Design review of the part shown in the three views and the two pictorial views. Dimensions are in mm from the part's minimum x, y and z. Give positions to 0.01 mm unless a question says otherwise; leave off trailing zeros. Order: outer loops, then holes, each group sorted by start corner. A loop starts at its lowest first (then second) coordinate and runs counter-clockwise, first axis right, second up. Notation, with made-up numbers: (20, 71.5) - (75, 71.5) arc R30 cw to (75, 103.5) - close; hole circle Ø9 at (36.5, 45.25). An arc over 180 degrees is marked (long way). Put each result on its own line as item: value.
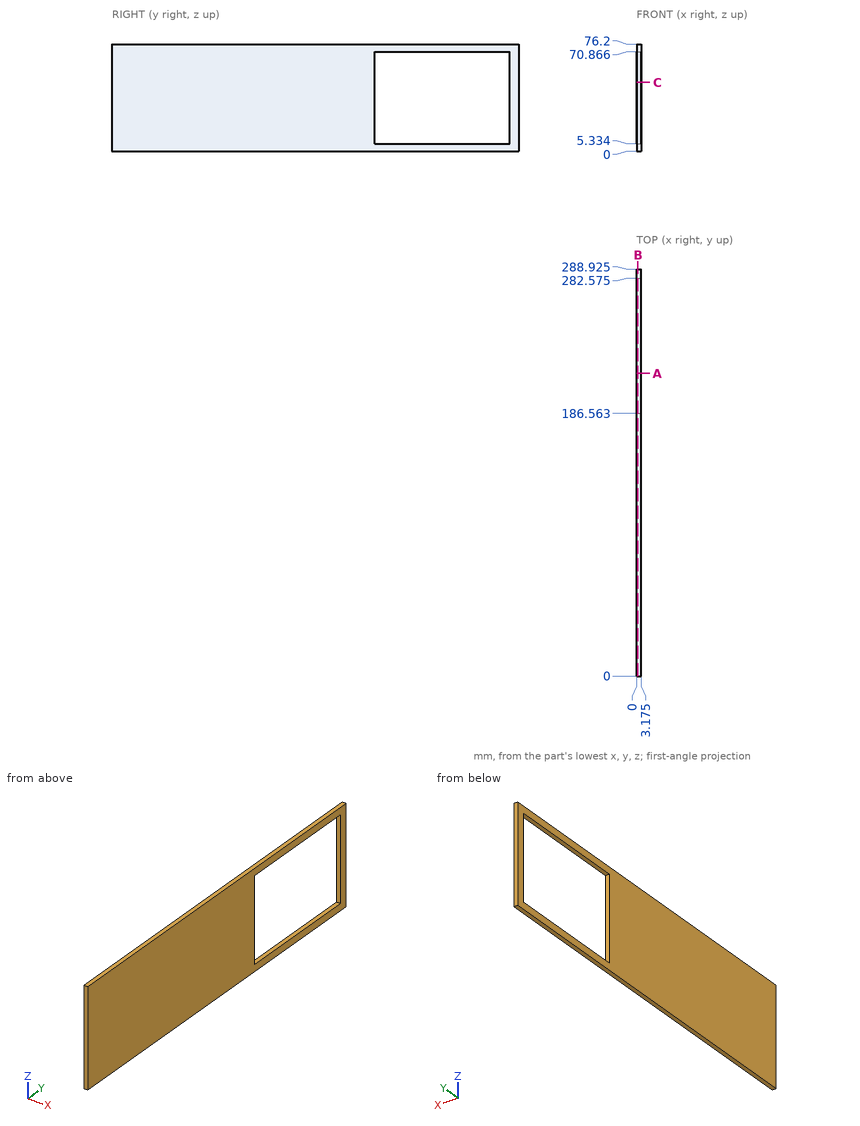
(1) Take a section at A-A, the plane y = 215. Write out the cut boundary in (x, z) (3 decimals), then the cut area to 3 significant figures.
The answers:
outline: (0, 0) - (3.175, 0) - (3.175, 5.334) - (0, 5.334) - close; (0, 70.866) - (3.175, 70.866) - (3.175, 76.2) - (0, 76.2) - close
area: 33.9 mm^2
(2) Take a section at B-B, the plane x = 0.9. Write out the cut boundary in (y, z) (3 decimals).
The answers:
outline: (0, 0) - (288.925, 0) - (288.925, 76.2) - (0, 76.2) - close; hole (186.563, 5.334) - (282.575, 5.334) - (282.575, 70.866) - (186.563, 70.866) - close
(3) Clearance check with a flat-ended pin moving along its axis: pin 1 Ø4 at (y, z) = (150, 11) entering from -X. State where the tip first meets the part, or that it passes through.
The answers:
pin 1: x = 0
(4) Take a section at C-C, the plane z = 49. Write out the cut boundary in (x, y) (3 decimals), then the cut area to 4 significant figures.
The answers:
outline: (0, 0) - (3.175, 0) - (3.175, 186.563) - (0, 186.563) - close; (0, 282.575) - (3.175, 282.575) - (3.175, 288.925) - (0, 288.925) - close
area: 612.5 mm^2
(5) Wall thickness on L1, parallel to Y at x = 0.45, z = 30 (3 decimals); L2, parallel to Z at x = 0.2, y = 267.5: over which ranges is each line inside the solid? List them lowest first.
The answers:
L1: 0 to 186.563, 282.575 to 288.925
L2: 0 to 5.33, 70.87 to 76.2
